Could you check a few things on this drawing? It's one solid part, dimensions in mm from its lowest x, y, z. A direction names the side the tool comes from. Give positions to 0.01 mm unless a question says otherwise; leave off trailing zeros. Order: outer loops, then holes, each group sorted by start corner. A loop starts at its lowest first (then second) coordinate and runs counter-clockwise, first axis right, second up. Notation, with made-up numbers: (86.5, 27.25) -> (96.5, 27.25) arc R18 ccw to (96.5, 60.25) -> close; hole circle Ø3 at (-19.75, -27). An arc over 180 degrees is marked (long way). Write each question's results on one line, items separated by ' | '.
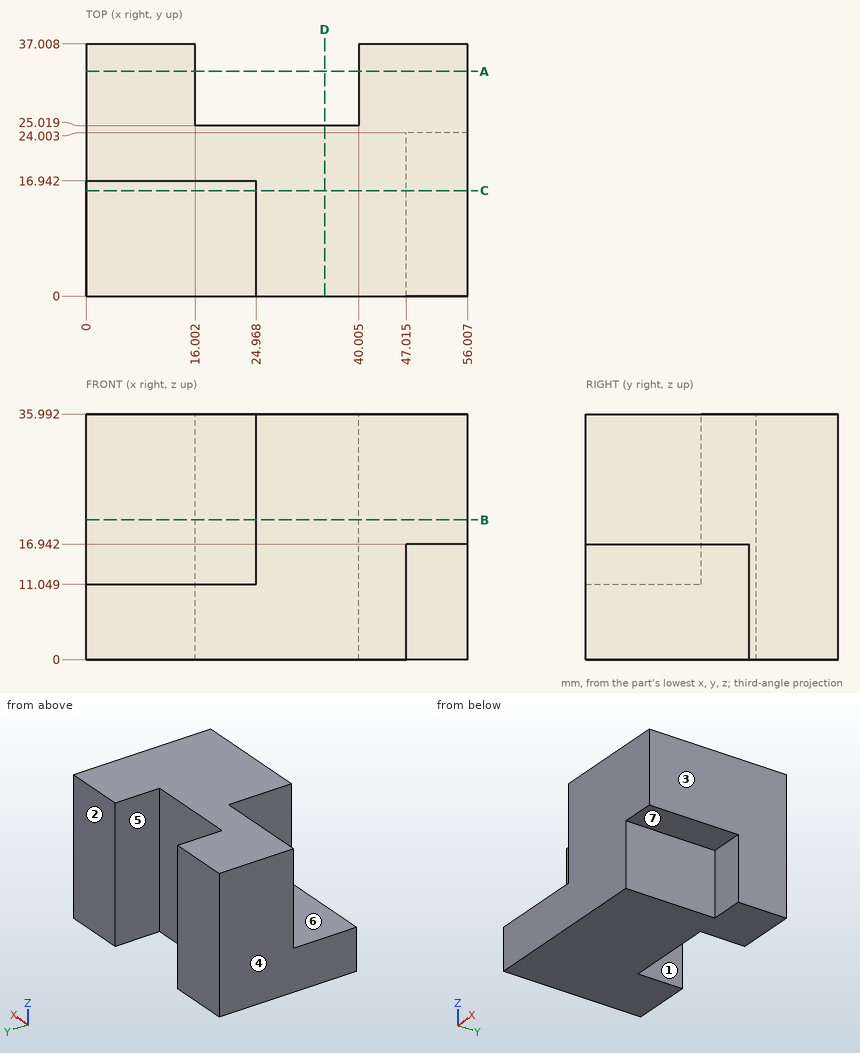
Q1. Suppose I cut it at A-A on y = 33. Please give me the cut outline in (x, z) (1 decimal).
Here are the results:
outline: (0, 0) -> (16, 0) -> (16, 36) -> (0, 36) -> close; (40, 0) -> (56, 0) -> (56, 36) -> (40, 36) -> close
Q2. I need wall thicknesses on line 1 along X through (y, z) = (32, 24) (1 decimal); line 2 along Y through (x, z) = (28, 34); line 3 along Y through (x, z) = (50, 10). Which ranges of each line are inside material? Lowest first, please.
Here are the results:
line 1: x = 0 to 16, 40 to 56 | line 2: y = 0 to 25.02 | line 3: y = 24 to 37.01
Q3. I'm going to push flat-ended pins straight in: pin 1 Ø13.5 at (y, z) = (16.5, 6.5) entering from +X (1 decimal); pin 2 Ø8.5 at (y, z) = (10.5, 25.5) entering from -X; pin 3 Ø12.5 at (x, z) = (12, 24.5) entering from -Y. Where does each tip first touch, or does it pass through?
Here are the results:
pin 1: stops at x = 47 | pin 2: stops at x = 24.97 | pin 3: stops at y = 16.94
Q4. Suppose I cut it at B-B on z = 20.5. Please give me the cut outline in (x, y) (1 decimal).
Here are the results:
outline: (0, 16.9) -> (25, 16.9) -> (25, 0) -> (56, 0) -> (56, 37) -> (40, 37) -> (40, 25) -> (16, 25) -> (16, 37) -> (0, 37) -> close
Q5. Thinking about a two-plate mould opening in X: for the marked faces 1, 2, 3 and 4, which applies, +X half, -X half, draft (parallel to the pull), parting line (faces both ways), or undercut?
Here are the results:
face 1: undercut | face 2: draft | face 3: +X half | face 4: -X half
Q6. For the marked faces 5, 6 and 7, which set-ups out of +Z, -Z, +X, -X, +Y, -Y let a thin tool reach every point of the face, with its end or its side?
Here are the results:
face 5: +Z, -Z, +Y | face 6: +Z, -X, -Y | face 7: -Z, +X, -Y
Q7. Suppose I cut it at D-D on x = 35. Please give me the cut outline in (y, z).
Here are the results:
outline: (0, 0) -> (25.02, 0) -> (25.02, 35.99) -> (0, 35.99) -> close
Q8. Suppose I cut it at C-C on y = 15.5. Please give me the cut outline in (x, z) (1 decimal), and give its area (3 significant figures).
Here are the results:
outline: (0, 0) -> (47, 0) -> (47, 16.9) -> (56, 16.9) -> (56, 36) -> (25, 36) -> (25, 11) -> (0, 11) -> close | area: 1,240 mm²
